from build123d import *

# Parameters (mm, degrees)
SKETCH2_W            = 60
SKETCH2_H            = 10
BOSS_EXTRUDE10_DEPTH = 50
BOSS_EXTRUDE11_DEPTH = 15
BOSS_EXTRUDE12_DEPTH = 35
BOSS_EXTRUDE14_DEPTH = 50
BOSS_EXTRUDE18_DEPTH = 35
SKETCH14_W           = 30
SKETCH14_H           = 10
CUT_EXTRUDE1_DEPTH   = 20


with BuildPart() as part:
    # Sketch2 → Boss-Extrude10 (new body)
    with BuildSketch(Plane.XY):
        with Locations((30, 5)):
            Rectangle(SKETCH2_W, SKETCH2_H)
    extrude(amount=BOSS_EXTRUDE10_DEPTH)

    # Sketch12 → Boss-Extrude14 (add)
    with BuildSketch(Plane.XY.offset(50)):
        with BuildLine():
            Line((30, 10), (60, 10))
            Line((60, 10), (60, 20))
            ThreePointArc((60, 20), (45.811388301, 12.565835097), (30, 10))
        make_face()
    extrude(amount=-BOSS_EXTRUDE14_DEPTH)



with BuildPart() as body_2:
    # Sketch9 → Boss-Extrude11 (new body)
    with BuildSketch(Plane(origin=(0, 0, 0), x_dir=(-1, 0, 0), z_dir=(0, 0, -1))):
        with BuildLine():
            Line((-30, 50), (-30, 20))
            Line((-30, 20), (0, 20))
            ThreePointArc((0, 20), (-8.786796564, 41.213203436), (-30, 50))
        make_face()
    extrude(amount=-BOSS_EXTRUDE11_DEPTH)

    # Sketch10 → Boss-Extrude12 (add)
    with BuildSketch(Plane(origin=(0, 0, 0), x_dir=(-1, 0, 0), z_dir=(0, 0, -1))):
        with BuildLine():
            Line((-60, 20), (-30, 20))
            Line((-30, 20), (-30, 50))
            ThreePointArc((-30, 50), (-51.213203436, 41.213203436), (-60, 20))
        make_face()
    extrude(amount=-BOSS_EXTRUDE12_DEPTH)


with BuildPart() as part_1:
    add(part.part)

    add(body_2.part)  # Boss-Extrude18 merges body 2
    # Sketch13 → Boss-Extrude18 (add)
    with BuildSketch(Plane(origin=(0, 0, 0), x_dir=(-1, 0, 0), z_dir=(0, 0, -1))):
        with BuildLine():
            Line((0, 20), (-60, 20))
            ThreePointArc((-60, 20), (-45.811388301, 12.565835097), (-30, 10))
            Line((-30, 10), (0, 10))
            Line((0, 10), (0, 20))
        make_face()
    extrude(amount=-BOSS_EXTRUDE18_DEPTH)

    # Sketch14 → Cut-Extrude1 (cut)
    with BuildSketch(Plane.XY.offset(35)):
        with Locations((15, 15)):
            Rectangle(SKETCH14_W, SKETCH14_H)
    extrude(amount=-CUT_EXTRUDE1_DEPTH, mode=Mode.SUBTRACT)


solid = part_1.part
Read the model definition and answer for the solid it produces. Units are mm, in the model's axes. A direction names the side the tool comes from. Round coordinates to 2 decimals unless told otherwise and drop trailing zeros. Write each loop counter-clockwise with the first axis right and the second up, starting at its lowest first coordinate (ties: lowest second). Pieces come first, ordered by that corner, then holes.
1. Which of the six approach directions +Z, -Z, +X, -X, +Y, -Y give full straight-line access (tool end or side, diameter ignored) to faces 1 (the face through (60, 10, 25)), 2 (the face through (15, 10, 33))?
2. The part is cut by section B-B, the plane y = 17. Determine the outline of the cut face in (x, z).
3. Straight lines are drawn through the part: L1, parallel to Y at x = 21, z = 38.5; L2, parallel to Z at x = 11, y = 30.5; L3, parallel to Z at x = 36.5, y = 38.5. For each, find the intervals that lie inside material, in ascending order.
4. Given pin 1 Ø9 at (x, y) = (46.5, 32.5) entering from +Z; pin 2 Ø6 at (y, z) = (37, 25) entering from -X; pin 3 Ø24 at (x, y) = (17, 33) entering from +Z, each flat-ended and moving along its own axis, determine where each tip first touches the part or whether it passes through.
5. The part is cut by section C-C, the plane x = 28. Determine the outline of the cut face in (y, z).
6. The part is cut by section A-A, the plane z = 23. Determine the outline of the cut face in (x, y).
7. The part is cut by section D-D, the plane z = 11.5. Determine the outline of the cut face in (x, y).
Values:
1. face 1: +Z, -Z, +X, +Y, -Y
1. face 2: +Z, -X, +Y
2. outline: (0, 0) - (60, 0) - (60, 50) - (55.51, 50) - (55.51, 35) - (30, 35) - (30, 15) - (0, 15) - close
3. L1: y = 0 to 10
3. L2: z = 0 to 15
3. L3: z = 0 to 35
4. pin 1: stops at z = 35
4. pin 2: stops at x = 30
4. pin 3: stops at z = 15
5. outline: (0, 0) - (49.93, 0) - (49.93, 15) - (10, 15) - (10, 50) - (0, 50) - close
6. outline: (0, 0) - (60, 0) - (60, 20) arc R30 ccw to (30, 50) - (30, 10) - (0, 10) - close
7. outline: (0, 0) - (60, 0) - (60, 20) arc R30 ccw to (0, 20) - close
